```python
from build123d import *

# Parameters (mm, degrees)
SKETCH1_W               = 38
SKETCH1_H               = 120
SKETCH1_W_2             = 21
SKETCH1_H_2             = 41
BOSS_EXTRUDE1_DEPTH     = 11
SKETCH3_R               = 1.3
CUT_EXTRUDE1_DEPTH      = 8
FILLET3_R               = 19
BOSS_EXTRUDE2_DEPTH     = 8
CUT_EXTRUDE2_DEPTH      = 66.741919656
CUT_EXTRUDE2_DEPTH_BACK = 66.741919656
SKETCH7_W               = 32
SKETCH7_H               = 50
BOSS_EXTRUDE4_DEPTH     = 8
SKETCH8_W               = 38
SKETCH8_H               = 50
BOSS_EXTRUDE5_DEPTH     = 8
BOSS_EXTRUDE10_START    = 2
SKETCH27_R              = 9
BOSS_EXTRUDE10_DEPTH    = 2
SKETCH28_W              = 38
SKETCH28_H              = 27
BOSS_EXTRUDE11_DEPTH    = 20
FILLET4_R               = 19
CUT_EXTRUDE14_DEPTH     = 8
CUT_EXTRUDE18_DEPTH     = 91.581455056
FILLET7_R               = 5
SKETCH35_R              = 1.1
CUT_EXTRUDE20_DEPTH     = 8
FILLET8_R               = 8
SKETCH36_R              = 6.45
CUT_EXTRUDE21_DEPTH     = 85.391942883
SKETCH30_W              = 13
SKETCH30_H              = 23
CUT_EXTRUDE22_DEPTH     = 13


# Some blends are built 0.0001 mm under size
with BuildPart() as part:
    # Sketch1 → Boss-Extrude1 (new body)
    with BuildSketch(Plane.XY):
        Rectangle(SKETCH1_W, SKETCH1_H)
        with Locations((0, -24.5)):
            Rectangle(SKETCH1_W_2, SKETCH1_H_2, mode=Mode.SUBTRACT)
    extrude(amount=BOSS_EXTRUDE1_DEPTH)

    # Sketch3 → Cut-Extrude1 (cut)
    with BuildSketch(Plane.XY.offset(10)):
        with Locations((-5, -0.5)):
            Circle(SKETCH3_R)
        with Locations((5, -0.5)):
            Circle(SKETCH3_R)
        with Locations((5, -48.5)):
            Circle(SKETCH3_R)
        with Locations((-5, -48.5)):
            Circle(SKETCH3_R)
    extrude(amount=-CUT_EXTRUDE1_DEPTH, mode=Mode.SUBTRACT)

    # Fillet3
    fillet3_edges = [part.edges().sort_by_distance(p)[0] for p in [
        (19, -60, 5.5),
        (-19, -60, 5.5),
    ]]
    fillet(fillet3_edges, radius=FILLET3_R - 0.0001)  # a hair under: the kernel refuses the full size

    # Sketch4 → Boss-Extrude2 (add)
    with BuildSketch(Plane.XY.offset(11)):
        with BuildLine():
            Line((19, -41), (19, 60))
            Line((19, 60), (-19, 60))
            Line((-19, 60), (-19, -41))
            ThreePointArc((-19, -41), (-13.435028843, -54.435028843), (0, -60))
            ThreePointArc((0, -60), (13.435028843, -54.435028843), (19, -41))
        make_face()
        with BuildLine():
            Line((16, -41), (16, 57))
            Line((16, 57), (-16, 57))
            Line((-16, 57), (-16, -41))
            ThreePointArc((-16, -41), (-11.313708499, -52.313708499), (0, -57))
            ThreePointArc((0, -57), (11.313708499, -52.313708499), (16, -41))
        make_face(mode=Mode.SUBTRACT)
    extrude(amount=BOSS_EXTRUDE2_DEPTH)

    # Sketch6 → Cut-Extrude2 (cut, two sides: drawn at the far end of the back side and taken through both)
    with BuildSketch(Plane(origin=(0, 0, 0), x_dir=(0, 0, -1), z_dir=(1, 0, 0)).offset(-CUT_EXTRUDE2_DEPTH_BACK)):
        Polygon((-13, -60), (-16, -35), (-19, -20), (-19, -60), align=None)
    extrude(amount=CUT_EXTRUDE2_DEPTH + CUT_EXTRUDE2_DEPTH_BACK, mode=Mode.SUBTRACT)

    # Sketch7 → Boss-Extrude4 (add)
    with BuildSketch(Plane.XY.offset(11)):
        with Locations((0, 32)):
            Rectangle(SKETCH7_W, SKETCH7_H)
    extrude(amount=BOSS_EXTRUDE4_DEPTH)

    # Sketch8 → Boss-Extrude5 (add)
    with BuildSketch(Plane(origin=(0, 0, 0), x_dir=(-1, 0, 0), z_dir=(0, 0, -1))):
        with Locations((0, 35)):
            Rectangle(SKETCH8_W, SKETCH8_H)
    extrude(amount=BOSS_EXTRUDE5_DEPTH)

    # Sketch27 → Boss-Extrude10 (add)
    with BuildSketch(Plane(origin=(0, 0, 0), x_dir=(-1, 0, 0), z_dir=(0, 0, -1)).offset(BOSS_EXTRUDE10_START)):
        with BuildLine():
            Line((19, -41), (19, 10))
            Line((19, 10), (-19, 10))
            Line((-19, 10), (-19, -41))
            ThreePointArc((-19, -41), (-13.435028843, -54.435028843), (0, -60))
            ThreePointArc((0, -60), (13.435028843, -54.435028843), (19, -41))
        make_face()
        with Locations((0, -34.75)):
            Circle(SKETCH27_R, mode=Mode.SUBTRACT)
    extrude(amount=-BOSS_EXTRUDE10_DEPTH)

    # Sketch28 → Boss-Extrude11 (add)
    with BuildSketch(Plane(origin=(0, 60, 0), x_dir=(1, 0, 0), z_dir=(0, 1, 0))):
        with Locations((0, -5.5)):
            Rectangle(SKETCH28_W, SKETCH28_H)
    extrude(amount=BOSS_EXTRUDE11_DEPTH)

    # Fillet4
    fillet4_edges = [part.edges().sort_by_distance(p)[0] for p in [
        (-19, 80, 5.5),
        (19, 80, 5.5),
    ]]
    fillet(fillet4_edges, radius=FILLET4_R - 0.0001)  # a hair under: the kernel refuses the full size

    # Sketch29 → Cut-Extrude14 (cut)
    with BuildSketch(Plane(origin=(0, 0, -8), x_dir=(-1, 0, 0), z_dir=(0, 0, -1))):
        with BuildLine():
            Line((16, 13), (16, 61))
            ThreePointArc((16, 61), (11.313708499, 72.313708499), (0, 77))
            ThreePointArc((0, 77), (-11.313708499, 72.313708499), (-16, 61))
            Line((-16, 61), (-16, 13))
            Line((-16, 13), (16, 13))
        make_face()
    extrude(amount=-CUT_EXTRUDE14_DEPTH, mode=Mode.SUBTRACT)

    # Sketch33 → Cut-Extrude18 (cut, through all)
    with BuildSketch(Plane(origin=(19, 0, 0), x_dir=(0, 0, -1), z_dir=(1, 0, 0))):
        Polygon((2, 80), (8, 40), (8, 80), align=None)
    extrude(amount=-CUT_EXTRUDE18_DEPTH, mode=Mode.SUBTRACT)

    # Fillet7
    # the kernel refuses this fillet: 5 mm, written as the material it takes off along each edge
    with BuildSketch(Plane(origin=(-19, 77.5, -8), x_dir=(0, 0, 1), z_dir=(0, -1, 0)), Plane(origin=(19, -2.5, -8), x_dir=(0, 0, 1), z_dir=(0, 1, 0))) as fillet7_piece_1:
        with BuildLine():
            CenterArc((FILLET7_R, -FILLET7_R), FILLET7_R, 90, 90)
            Line((0, -FILLET7_R), (0, 0))
            Line((0, 0), (FILLET7_R, 0))
        make_face()
    extrude(amount=80, mode=Mode.SUBTRACT)
    with BuildSketch(Plane(origin=(-19, -57.5, 19), x_dir=(1, 0, 0), z_dir=(0, 1, 0)), Plane(origin=(19, 61.0001, 19), x_dir=(-1, 0, 0), z_dir=(0, -1, 0))) as fillet7_piece_2:
        with BuildLine():
            CenterArc((FILLET7_R, FILLET7_R), FILLET7_R, 180, 90)
            Line((0, FILLET7_R), (0, 0))
            Line((0, 0), (FILLET7_R, 0))
        make_face()
    extrude(amount=118.5001, mode=Mode.SUBTRACT)
    with BuildSketch(Plane(origin=(0.0001, 61.0001, 19), x_dir=(0, 1, 0), z_dir=(-1, 0, 0))) as fillet7_piece_3:
        with BuildLine():
            CenterArc((18.9999 - FILLET7_R, FILLET7_R), FILLET7_R, 270, 90)
            Line((18.9999, FILLET7_R), (18.9999, 0))
            Line((18.9999, 0), (18.9999 - FILLET7_R, 0))
        make_face()
    revolve(axis=Axis((0.0001, 61.0001, 19), (0, 0, -1)), revolution_arc=90, mode=Mode.SUBTRACT)
    with BuildSketch(Plane(origin=(-0.0001, 61.0001, 19), x_dir=(0, 1, 0), z_dir=(1, 0, 0))) as fillet7_piece_4:
        with BuildLine():
            CenterArc((18.9999 - FILLET7_R, -FILLET7_R), FILLET7_R, 0, 90)
            Line((18.9999, -FILLET7_R), (18.9999, 0))
            Line((18.9999, 0), (18.9999 - FILLET7_R, 0))
        make_face()
    revolve(axis=Axis((-0.0001, 61.0001, 19), (0, 0, 1)), revolution_arc=90, mode=Mode.SUBTRACT)
    with BuildSketch(Plane(origin=(-0.0001, 80, 19), x_dir=(0, -1, 0), z_dir=(1, 0, 0))) as fillet7_piece_5:
        with BuildLine():
            CenterArc((FILLET7_R, FILLET7_R), FILLET7_R, 180, 90)
            Line((0, FILLET7_R), (0, 0))
            Line((0, 0), (FILLET7_R, 0))
        make_face()
    extrude(amount=0.0002, mode=Mode.SUBTRACT)

    # Sketch35 → Cut-Extrude20 (cut)
    with BuildSketch(Plane.XY.offset(11)):
        with Locations((-5, -0.5)):
            Circle(SKETCH35_R)
        with Locations((5, -0.5)):
            Circle(SKETCH35_R)
        with Locations((5, -48.5)):
            Circle(SKETCH35_R)
        with Locations((-5, -48.5)):
            Circle(SKETCH35_R)
    extrude(amount=-CUT_EXTRUDE20_DEPTH, mode=Mode.SUBTRACT)

    # Fillet8
    fillet8_edges = [part.edges().sort_by_distance(p)[0] for p in [
        (-16, 7, 14.791287847),
        (16, 7, 14.791287847),
        (16, 13, -3.791287847),
        (-16, 13, -3.791287847),
    ]]
    fillet(fillet8_edges, radius=FILLET8_R)

    # Sketch36 → Cut-Extrude21 (cut, through all)
    with BuildSketch(Plane(origin=(0, 0, 0), x_dir=(-1, 0, 0), z_dir=(0, 0, -1))):
        with Locations((1.882410705, 50.832111393)):
            Circle(SKETCH36_R)
    extrude(amount=-CUT_EXTRUDE21_DEPTH, mode=Mode.SUBTRACT)

    # Sketch30 → Cut-Extrude22 (cut)
    with BuildSketch(Plane(origin=(0, 0, 0), x_dir=(-1, 0, 0), z_dir=(0, 0, -1))):
        with Locations((1.882410705, 46)):
            Rectangle(SKETCH30_W, SKETCH30_H)
    extrude(amount=-CUT_EXTRUDE22_DEPTH, mode=Mode.SUBTRACT)


solid = part.part
```
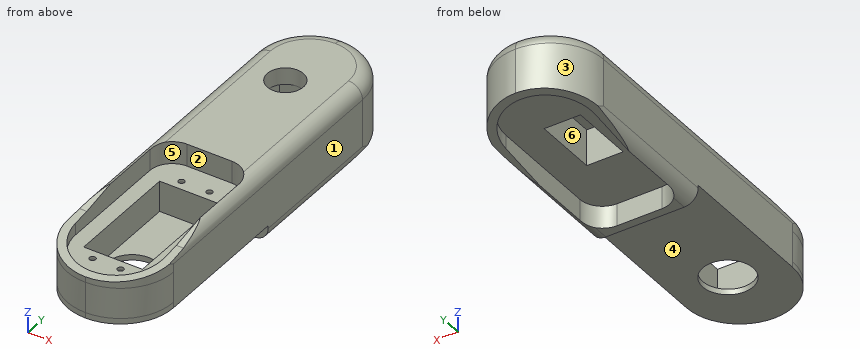
Work out the finished part from the listing and answer in its coordinate system (mm). Face numbers are marked on the shaded views. A direction names the side the tool comes from. Give positions to 0.01 mm unless a question says otherwise; leave off trailing zeros. Loops run counter-clockwise (first coordinate to the right, second up) from the corner with the lowest first, then second, coordinate; pieces in that order, holes last. Notation, with made-up numbers: (79.5, -17.75) -> (83.5, -17.75) arc R14 cw to (83.5, -7.75) -> close; hole circle Ø4 at (-23.75, 29). An arc over 180 degrees is marked (long way). Put each result on its own line as item: value. Start each with the question number.
Item 1: The part is cut by section B-B (y = -30.5). Give the vertices of the cut face in (x, z), then the cut area to 3 significant figures.
Item 2: The part is cut by section C-C (y = 59). Give the vertices of the cut face in (x, z).
Item 3: Each of these flat-tipped pins is pushed along its axis until it touches: P1, Ø20.5, axis at x = 0, y = -34.75, coming from the -Z side; P2, Ø4, axis at x = 3, z = 13.5, coming from the -Y side; P3, Ø2.5, axis at y = 34, z = -5.5, coming from the +X side. Where does it stop, or does it pass through?
Item 4: Which of the six approach directions +Z, -Z, +X, -X, +Y, -Y give full straight-line access (tool end or side, diameter ignored) to the marked faces 4, 5 and 6?
Item 5: The mould has two halves that part along Y. Classify the marked faces 1, 2 and 3: released by +Y, released by -Y, zero draft, split by the parting line, or undercut.
Item 6: The part is cut by section A-A (z = 8.25). State how many separate pieces and enclosed holes the cut face has, then the cut area to 3 significant figures.
Item 7: Find the intervals of material crossed by L1, parallel to Y at x = 0, z = -1.35; L2, parallel to X at y = -9, z = 6.75; L3, parallel to Y at x = -5, z = 5.25, in increasing order. Write a range as [from, to].
Answers below:
1. outline: (-19, -2) -> (-7.93, -2) -> (-7.93, 0) -> (-10.5, 0) -> (-10.5, 11) -> (-16, 11) -> (-16, 16.9) -> (-18.07, 16.9) arc R5 ccw to (-19, 14) -> close; (7.93, -2) -> (19, -2) -> (19, 14) arc R5 ccw to (18.07, 16.9) -> (16, 16.9) -> (16, 11) -> (10.5, 11) -> (10.5, 0) -> (7.93, 0) -> close
1. area: 265 mm2
2. outline: (-19, -3) arc R5 ccw to (-18.51, -5.15) -> (-16, -5.15) -> (-16, 0) -> (16, 0) -> (16, -5.15) -> (18.51, -5.15) arc R5 ccw to (19, -3) -> (19, 14) arc R5 ccw to (14, 19) -> (-14, 19) arc R5 ccw to (-19, 14) -> close
3. P1: z = -2
3. P2: y = -59.97
3. P3: x = 18.84
4. face 4: -Z, +X, -X, -Y
4. face 5: +Z
4. face 6: -Z
5. face 1: zero draft
5. face 2: undercut
5. face 3: released by +Y
6. separate pieces: 1
6. enclosed holes: 6
6. area: 3,830 mm2
7. L1: [-60, -43.75], [-25.75, 13], [77, 80]
7. L2: [-19, -10.5], [10.5, 19]
7. L3: [-59.33, -49.8], [-47.2, -45], [-4, -1.8], [0.8, 34.5], [57.5, 79.33]
